Work out the finished part from the listing and answer in its coordinate system (mm). Face numbers are marked on the shaded views. A direction names the side the tool comes from. Give positions to 0.01 mm unless a question says otherwise; leave off trailing zeros. Order: outer loops, then holes, each group sorted by start corner. A loop starts at its lowest first (then second) coordinate and runs counter-clockwise, first axis right, second up. Notation, with made-up numbers: M 30.5,32.5 L 55.5,32.5 A11 cw 55.5,45.5 Z; hole C 58,38 d9. An arc over 180 degrees is marked long. One line per item, written item: value.
from build123d import *

# Parameters (mm, degrees)
SKETCH_1_W      = 27
SKETCH_1_H      = 12
SKETCH_1_W_2    = 23
SKETCH_1_H_2    = 9
EXTRUDE_1_DEPTH = 8
SKETCH_2_W      = 11
SKETCH_2_H      = 9
EXTRUDE_2_DEPTH = 2
SKETCH_3_R      = 2.75
SKETCH_3_R_2    = 1.55
EXTRUDE_3_DEPTH = 5


with BuildPart() as part:
    # 草图1 → 凸台-拉伸1 (new body)
    with BuildSketch(Plane.XY):
        Rectangle(SKETCH_1_W, SKETCH_1_H)
        Rectangle(SKETCH_1_W_2, SKETCH_1_H_2, mode=Mode.SUBTRACT)
    extrude(amount=EXTRUDE_1_DEPTH)

    # 草图2 → 凸台-拉伸2 (add)
    with BuildSketch(Plane.XY.offset(8)):
        with Locations((6, 0)):
            Rectangle(SKETCH_2_W, SKETCH_2_H)
    extrude(amount=-EXTRUDE_2_DEPTH)

    # 草图3 → 凸台-拉伸3 (add)
    with BuildSketch(Plane(origin=(0, 0, 6), x_dir=(-1, 0, 0), z_dir=(0, 0, -1))):
        with Locations((-6.35, 0)):
            Circle(SKETCH_3_R)
        with Locations((-6.35, 0)):
            Circle(SKETCH_3_R_2, mode=Mode.SUBTRACT)
    extrude(amount=EXTRUDE_3_DEPTH)


solid = part.part
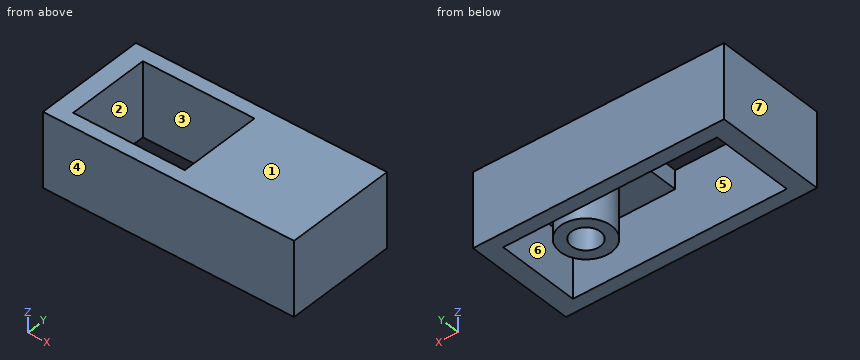
(1) Given P1, Ø4.5, axis at x = 8.5, y = -2, coming from the -Z side, flat-ended and moving along its own axis, determine where the tip first touches the part or whether it passes through.
Findings:
P1: stops at z = 1
(2) Section A-A, the plane z = 1.5 is taken. Give the vertices of the cut face in (x, y), then the cut area to 3 significant figures.
Findings:
outline: M -13.5,-6 L 13.5,-6 L 13.5,6 L -13.5,6 Z; C 6.35,0 d5.5; hole M -11.5,-4.5 L 11.5,-4.5 L 11.5,4.5 L -11.5,4.5 Z; hole C 6.35,0 d3.1
area: 133 mm^2
(3) Section D-D, the plane x = 2.75 is taken. Give the vertices of the cut face in (y, z).
Findings:
outline: M -6,0 L -4.5,0 L -4.5,6 L 4.5,6 L 4.5,0 L 6,0 L 6,8 L -6,8 Z
(4) Section C-C, the plane y = 0 is taken. Give the vertices of the cut face in (x, z), then the cut area to 3 significant figures.
Findings:
outline: M -13.5,0 L -11.5,0 L -11.5,8 L -13.5,8 Z; M 0.5,6 L 3.6,6 L 3.6,1 L 4.8,1 L 4.8,6 L 7.9,6 L 7.9,1 L 9.1,1 L 9.1,6 L 11.5,6 L 11.5,0 L 13.5,0 L 13.5,8 L 0.5,8 Z
area: 66.0 mm^2
(5) Section B-B, the plane x = -2.5 is taken. Give the vertices of the cut face in (y, z).
Findings:
outline: M -6,0 L -4.5,0 L -4.5,8 L -6,8 Z; M 4.5,0 L 6,0 L 6,8 L 4.5,8 Z
(6) Find the intervals of material crossed by probe 1 along Y at (x, z) = (6.35, 3.35); probe 2 along X at (y, z) = (-1.75, 4.5); probe 3 along X at (y, z) = (-2.5, 5.25), in increasing order. Write a range as from..to.
Findings:
probe 1: y = -6..-4.5, -2.75..-1.55, 1.55..2.75, 4.5..6
probe 2: x = -13.5..-11.5, 4.23..8.47, 11.5..13.5
probe 3: x = -13.5..-11.5, 5.2..7.5, 11.5..13.5
(7) Which of the six approach directions +Z, -Z, +X, -X, +Y, -Y give full straight-line access (tool end or side, diameter ignored) to the marked faces 1, 2 and 3?
Findings:
face 1: +Z, +X, -X, +Y, -Y
face 2: +Z, -Z
face 3: -Z
(8) Determine the mould class of the marked faces 4, 5, 6 and 7 for opening direction Y: pulls with the +Y half, pulls with the -Y half, needs draft (parallel to the pull), parting line crosses it, or undercut.
Findings:
face 4: pulls with the -Y half
face 5: undercut
face 6: undercut
face 7: needs draft
